The model under review builds one solid part; all positions refer to its coordinate system, in mm. A direction names the side the tool comes from. Round coordinates to 2 decimals unless told otherwise and drop trailing zeros. Write each loop counter-clockwise with the first axis right and the second up, starting at its lowest first coordinate (ties: lowest second). Pieces come first, ordered by that corner, then holes. Notation, with made-up numbers: (-15, 77.5) -> (42, 77.5) arc R20 ccw to (42, 96.5) -> close; hole circle Ø9 at (60.25, 87.25). An arc over 180 degrees is marked (long way). Use CSV: the item, a comma, the result in double quotes. Start each with the question number.
1) Take a section at A-A, the plane x = 12.7. Give the boundary of the cut face in (y, z), then the cut area to 3 significant figures.
2) Wall thickness on probe 1 along Z at (x, y) = (12.7, -21); probe 2 along Y at (x, z) = (10, 14); probe 3 along Z at (x, y) = (17.5, -16.25): over which ranges is each line inside the solid? List them lowest first. Write a range as [from, to].
3) Take a section at C-C, the plane x = 9. Give the boundary of the cut face in (y, z).
4) Take a section at B-B, the plane z = 12.5. Give the boundary of the cut face in (x, y).
5) Machinability: for faces 1 (the face through (15, -21.954, 12)), 2 (the face through (12.5, -5.6, 18.693)), which of the approach directions +Z, -Z, +X, -X, +Y, -Y give a long, thin tool a straight path to every point of the face, cutting with its end or side? Answer none if there is none.
6) Take a section at D-D, the plane y = -5.5. Give the boundary of the cut face in (x, z).
7) For pin 1 Ø8 at (x, z) = (3, 5) entering from +Y; pin 2 Ø1.5 at (x, y) = (13.5, -1.5) entering from -Z; pin 3 Ø2 at (y, z) = (-2, 18.5) entering from -X, all flat-tipped, find the tip position at first contact; note any pin that passes through.
8) Mouldability with a two-part tool opening along Y and no side actions: class faces 3 (the face through (13, 3.446, 20)), 4 (the face through (10.18, -11.186, 19.981)), 5 (the face through (13, -21, -4.167)) as released by +Y, released by -Y, zero draft, split by the parting line, or undercut.
Autodesk Inventor part; units mm, degrees
ref_plane "YZ Plane" through (0, 0, 0) normal (1, 0, 0) x (0, 1, 0)
ref_plane "XZ Plane" through (0, 0, 0) normal (0, 1, 0) x (-1, 0, 0)
ref_plane "XY Plane" through (0, 0, 0) normal (0, 0, 1) x (1, 0, 0)
sketch "Sketch1" plane through (0, 0, 0) normal (1, 0, 0) x (0, 1, 0)
  line L0 (-21.9539, 18.6933) -> (3.4461, 18.6933)
  line L1 (3.4461, 18.6933) -> (3.4461, 21.2333)
  line L2 (3.4461, 21.2333) -> (-21.9539, 21.2333)
  line L3 (-21.9539, 21.2333) -> (-21.9539, 18.6933)
  line L4 (-21.9539, 18.6933) -> (-19.4139, 18.6933)
  line L5 (-19.4139, 18.6933) -> (-19.4139, -4.1667)
  line L6 (-19.4139, -4.1667) -> (-21.9539, -4.1667)
  line L7 (-21.9539, -4.1667) -> (-21.9539, 18.6933)
  point P0 (0, 0)
  dimension "d0" = 2.54
  dimension "d1" = 2.54
  dimension "d2" = 25.4
  dimension "d3" = 25.4
extrude "Extrusion1" add sketch "Sketch1" along normal blind 25.4
sketch "Sketch2" plane through (0, -21.9539, 21.2333) normal (0, 0, 1) x (1, 0, 0)
  circle A0 centre (12.7, 12.7) radius 3.175
  line L0 (0, 25.4) -> (25.4, 25.4)
  line L1 (25.4, 25.4) -> (25.4, 0)
  point P0 (0, 21.9539)
  dimension "d6" = 6.35
  dimension "d7" = 12.7
  dimension "d8" = 12.7
extrude "Extrusion2" cut sketch "Sketch2" against normal blind 25.4
sketch "Sketch3" plane through (0, -21.9539, -4.1667) normal (0, -1, 0) x (1, 0, 0)
  circle A0 centre (12.7, 12.7) radius 3.175
  line L0 (0, 25.4) -> (25.4, 25.4)
  line L1 (25.4, 25.4) -> (25.4, 0)
  point P0 (0, 4.1667)
  dimension "d11" = 12.7
  dimension "d12" = 12.7
  dimension "d13" = 6.35
extrude "Extrusion3" cut sketch "Sketch3" against normal blind 25.4
fillet "Fillet1" radius 7.62 4 edges at (25.4, 3.4461, 19.9633) (0, 3.4461, 19.9633) (25.4, -20.6839, -4.1667) (0, -20.6839, -4.1667)
properties part number "80-20 bracket 1in"
Values found:
1,outline,"(-21.95, -4.17) -> (-19.41, -4.17) -> (-19.41, 5.36) -> (-21.95, 5.36) -> close; (-21.95, 11.71) -> (-19.41, 11.71) -> (-19.41, 18.69) -> (-12.43, 18.69) -> (-12.43, 21.23) -> (-21.95, 21.23) -> close; (-6.08, 18.69) -> (3.45, 18.69) -> (3.45, 21.23) -> (-6.08, 21.23) -> close"
1,area,"90.3 mm²"
2,probe 1,"[-4.17, 5.36], [11.71, 21.23]"
2,probe 2,"[-21.95, -19.41]"
2,probe 3,"[18.69, 21.23]"
3,outline,"(-21.95, -4.17) -> (-19.41, -4.17) -> (-19.41, 18.69) -> (3.45, 18.69) -> (3.45, 21.23) -> (-21.95, 21.23) -> close"
4,outline,"(0, -21.95) -> (25.4, -21.95) -> (25.4, -19.41) -> (0, -19.41) -> close"
5,face 1,"+Z, -Z, +X, -X, -Y"
5,face 2,"-Z, +X, -X, +Y"
6,outline,"(0, 18.69) -> (25.4, 18.69) -> (25.4, 21.23) -> (0, 21.23) -> close"
7,pin 1,"y = -19.41"
7,pin 2,"z = 18.69"
7,pin 3,"x = 0.09"
8,face 3,"released by +Y"
8,face 4,"undercut"
8,face 5,"zero draft"
